from build123d import *

# Parameters (mm, degrees)
F1_DEPTH = 3
F2_DEPTH = 25
F3_DEPTH = 25


with BuildPart() as f1:
    # F0 (on Top) → F1 (new body)
    with BuildSketch(Plane.XY):
        with BuildLine():
            Line((0, 141.9), (0, 147))
            Line((0, 147), (-134.61055, 147))
            ThreePointArc((-134.61055, 147), (-136.772472, 136.772472), (-147, 134.61055))
            Line((-147, 134.61055), (-147, 0))
            Line((-147, 0), (-142, 0))
            Line((-142, 0), (-145, 20))
            Line((-145, 20), (-130, 20))
            Line((-130, 20), (-133, 0))
            Line((-133, 0), (-125, 0))
            Line((-125, 0), (-125, 125))
            Line((-125, 125), (0, 125))
            Line((0, 125), (0, 133.1))
            Line((0, 133.1), (20, 130.1))
            Line((20, 130.1), (20, 144.9))
            Line((20, 144.9), (0, 141.9))
        make_face()
    extrude(amount=F1_DEPTH)

    # F0 (on Top) → F2 (join)
    with BuildSketch(Plane.XY):
        with BuildLine():
            ThreePointArc((-147, 137.61055), (-148.90564, 139.395179), (-150, 141.765568))
            Line((-150, 141.765568), (-150, 0))
            Line((-150, 0), (-147, 0))
            Line((-147, 0), (-147, 134.61055))
            Line((-147, 134.61055), (-147, 137.61055))
        make_face()
        with BuildLine():
            Line((0, 150), (-141.765568, 150))
            ThreePointArc((-141.765568, 150), (-139.395179, 148.90564), (-137.61055, 147))
            Line((-137.61055, 147), (-134.61055, 147))
            Line((-134.61055, 147), (0, 147))
            Line((0, 147), (0, 150))
        make_face()
    extrude(amount=F2_DEPTH)

    # F0 (on Top) → F3 (join)
    with BuildSketch(Plane.XY):
        with BuildLine():
            Line((-134.61055, 147), (-137.61055, 147))
            ThreePointArc((-137.61055, 147), (-138.565994, 138.565994), (-147, 137.61055))
            Line((-147, 137.61055), (-147, 134.61055))
            ThreePointArc((-147, 134.61055), (-136.772472, 136.772472), (-134.61055, 147))
        make_face()
    extrude(amount=F3_DEPTH)


solid = f1.part
For this review, take the finished solid that the model builds, in its own axes (mm). Give positions to 0.01 mm unless a question says otherwise; leave off trailing zeros. Loops run counter-clockwise (first coordinate to the right, second up) from the corner with the lowest first, then second, coordinate; pieces in that order, holes last.
Item 1: Take a section at A-A, the plane x = -102. State the section outline as (y, z) points, and give its area (3 significant figures).
Item 2: Take a section at B-B, the plane y = 32. State the section outline as (x, z) points, and give its area (3 significant figures).
Item 3: Draft analysis for pull direction X (two halves, no side actions). For faces 1 (the flat face through (-126, 101, 3)), 2 (the flat face through (-150, 72, 12)), 3 (the cylindrical face through (-136.883, 136.664, 13.846)), state which applies: +X half, -X half, draft (parallel to the pull), parting line (faces both ways), or undercut.
Item 4: Insertion check: pin 1 (0.9 mm diameter, centred on x = -140, z = 1, fed in from -Y); pin 2 (2 mm diameter, centred on y = 106.5, z = 19.5, fed in from +X); pin 3 (2.5 mm diameter, centred on x = -93.5, z = 1.5, fed in from -Y); pin 4 (0.9 mm diameter, centred on y = 130, z = 1.5, fed in from +X). Each pin has a flat end and moves straight along its axis. Give the tip position at first contact, or say it passes through.
Item 5: For line 1 along X through (y, z) = (12.5, 12.25); line 2 along Z through (x, y) = (9.5, 133.5); line 3 along Y through (x, z) = (-114, 6.75), list the stretches that pass through material, from the lowest coordinate up.
Item 6: Take a section at C-C, the plane z = 17.75. State the section outline as (x, y) points.
Calculated:
1. outline: (125, 0) - (150, 0) - (150, 25) - (147, 25) - (147, 3) - (125, 3) - close
1. area: 141 mm2
2. outline: (-150, 0) - (-125, 0) - (-125, 3) - (-147, 3) - (-147, 25) - (-150, 25) - close
2. area: 141 mm2
3. face 1: draft
3. face 2: -X half
3. face 3: undercut
4. pin 1: stops at y = 20
4. pin 2: stops at x = -147
4. pin 3: stops at y = 125
4. pin 4: stops at x = 20
5. line 1: x = -150 to -147
5. line 2: z = 0 to 3
5. line 3: y = 147 to 150
6. outline: (-150, 0) - (-147, 0) - (-147, 134.61) arc R9.58 ccw to (-134.61, 147) - (0, 147) - (0, 150) - (-141.77, 150) arc R6.81 cw to (-137.61, 147) arc R6.81 cw to (-147, 137.61) arc R6.81 cw to (-150, 141.77) - close
